from build123d import *

# Parameters (mm, degrees)
CROQUIS1_W              = 55
CROQUIS1_H              = 12
SALIENTE_EXTRUIR1_DEPTH = 12
TALADRO1_OUTLINE_R      = 2.5
TALADRO1_DEPTH          = 12


# Read off the part's stored shape, not the designer's step: Taladro1
with BuildPart() as part:
    # Croquis1 → Saliente-Extruir1 (new body)
    with BuildSketch(Plane.XY):
        with Locations((27.5, 6)):
            Rectangle(CROQUIS1_W, CROQUIS1_H)
        with BuildLine():
            ThreePointArc((27.5, 9), (18.5, 6), (27.5, 3))
            ThreePointArc((27.5, 3), (36.5, 6), (27.5, 9))
        make_face(mode=Mode.SUBTRACT)
    extrude(amount=SALIENTE_EXTRUIR1_DEPTH)

    # Taladro1 outline → Taladro1 (cut)
    with BuildSketch(Plane(origin=(0, 0, 0), x_dir=(1, 0, 0), z_dir=(0, 1, 0))):
        with Locations((48, -6)):
            Circle(TALADRO1_OUTLINE_R)
        with Locations((7, -6)):
            Circle(TALADRO1_OUTLINE_R)
    extrude(amount=TALADRO1_DEPTH, mode=Mode.SUBTRACT)


solid = part.part
Can you work these out from the model? Positions are in its coordinate system, mm. Round coordinates to 2 decimals unless told otherwise and drop trailing zeros. Write each loop counter-clockwise with the first axis right and the second up, starting at its lowest first coordinate (ties: lowest second). Pieces come first, ordered by that corner, then holes. Notation, with made-up numbers: M 85.25,-25 L 138.25,-25 A29 ccw 138.25,9 Z; hole C 52,24 d11. An arc over 180 degrees is marked long. Use CSV: the item, a comma, the result in double quotes.
(1) Imagine slicing it at D-D (y = 6). Write out the boundary of the cut face in (x, z), plus the area to 3 significant figures.
Check values:
outline,"M 0,0 L 18.5,0 L 18.5,12 L 0,12 Z; M 36.5,0 L 55,0 L 55,12 L 36.5,12 Z; hole C 7,6 d5; hole C 48,6 d5"
area,"405 mm^2"
(2) Imagine slicing it at A-A (y = 2). Write out the boundary of the cut face in (x, z), plus the area to 3 significant figures.
Check values:
outline,"M 0,0 L 20.5,0 L 20.5,12 L 0,12 Z; M 26.5,0 L 28.5,0 L 28.5,12 L 26.5,12 Z; M 34.5,0 L 55,0 L 55,12 L 34.5,12 Z; hole C 7,6 d5; hole C 48,6 d5"
area,"477 mm^2"
(3) We'd pull the mould along X, two halves only. Please class faces 1 (the flat face through (27, 10, 0)), 2 (the cylindrical face through (50.31, 5.92, 6.96)), 3 (the flat face through (0, 6, 6)), 4 (the cylindrical face through (36.497, 5.825, 5.916)): +X half, -X half, draft (parallel to the pull), parting line (faces both ways), or undercut.
Check values:
face 1,"draft"
face 2,"undercut"
face 3,"-X half"
face 4,"undercut"
(4) Imagine slicing it at C-C (x = 5). Write out the boundary of the cut face in (y, z).
Check values:
outline,"M 0,0 L 12,0 L 12,4.5 L 0,4.5 Z; M 0,7.5 L 12,7.5 L 12,12 L 0,12 Z"
(5) I need wall thicknesses on line 1 along X through (y, z) = (6.25, 6); line 2 along X through (y, z) = (6, 9.25); line 3 along Z through (x, y) = (48, 5). Which ranges of each line are inside material? Lowest first, please.
Check values:
line 1,"0 to 4.5, 9.5 to 18.51, 36.49 to 45.5, 50.5 to 55"
line 2,"0 to 18.5, 36.5 to 55"
line 3,"0 to 3.5, 8.5 to 12"
(6) Imagine slicing it at B-B (z = 4.5). Write out the boundary of the cut face in (x, y).
Check values:
outline,"M 0,0 L 5,0 L 5,12 L 0,12 Z; M 9,0 L 46,0 L 46,12 L 9,12 Z; M 50,0 L 55,0 L 55,12 L 50,12 Z; hole M 27.5,3 A5 ccw long 27.5,9 A5 ccw long Z"
